Autodesk Inventor part; units mm, degrees
ref_plane "YZ Plane" through (0, 0, 0) normal (1, 0, 0) x (0, 1, 0)
ref_plane "XZ Plane" through (0, 0, 0) normal (0, 1, 0) x (-1, 0, 0)
ref_plane "XY Plane" through (0, 0, 0) normal (0, 0, 1) x (1, 0, 0)
sketch "スケッチ1" plane through (0, 0, 0) normal (1, 0, 0) x (0, 1, 0)
  line L0 (0, 0) -> (1.25, 0)
  line L1 (1.25, 0) -> (1.25, -10)
  line L2 (1.25, -10) -> (0, -10)
  line L3 (0, -10) -> (0, 0)
  line L4 (0, -10) -> (2.25, -10)
  line L5 (2.25, -10) -> (2.25, -12.5)
  line L6 (2.25, -12.5) -> (0, -12.5)
  line L7 (0, -12.5) -> (0, -10)
  line L8 (2.25, -12.3) -> (2.05, -12.5)
  line L9 (1.25, -0.12) -> (1.13, 0)
  point P0 (2.25, -11.25)
  point P1 (1.25, -10)
  dimension "d0" = 45
  dimension "d1" = 2.25
  dimension "d2" = 2.5
  dimension "d3" = 10
  dimension "d7" = 1.25
  dimension "d10" = 45
  dimension "d11" = 0.2
  dimension "d12" = 0.12
revolve "回転1" add sketch "スケッチ1" angle 360 about axis through (0, 0, -10) along (0, 0, 1) contours L0 L9 L1 L2 L3 | L2 L4 L5 L8 L6 L7
thread "ねじ2"
properties part number "CSH-316L-M2_5-10" material "ステンレス鋼"
CAD build for the part. Positions are in the model's coordinates, mm. A direction names the side the tool comes from. Coordinates: 2 decimals unless noted, no trailing zeros. Order: outer loops, then holes, each group sorted by start corner. A loop starts at its lowest first (then second) coordinate and runs counter-clockwise, first axis right, second up. Notation, with made-up numbers: (-2, -34) - (32, -34) arc R16 cw to (32, -14) - close; hole circle Ø6 at (-12, 20.5). An arc over 180 degrees is marked (long way). Answer in a Markdown table with one row per item.
1. 3-axis set-ups, long thin cutter, end or side, ignore diameter. For faces 3 (the face through (0, 0, -12.5)), 4 (the face through (-1.22, -0.27, -5.13)): which of +Z, -Z, +X, -X, +Y, -Y reach the whole face in a straight line?
Answer:
| item | result |
|---|---|
| face 3 | -Z, +X, -X, +Y, -Y |
| face 4 | +Z |
2. Slice it at C-C, the plane z = -5.75. List the corners of the cut face in (x, y), then the cut area to 3 significant figures.
Answer:
| item | result |
|---|---|
| outline | circle Ø2.5 at (0, 0) |
| area | 4.91 mm² |
3. Slice it at A-A, the plane x = 0. List the corners of the cut face in (y, z).
Answer:
| item | result |
|---|---|
| outline | (-2.25, -12.3) - (-2.05, -12.5) - (2.05, -12.5) - (2.25, -12.3) - (2.25, -10) - (1.25, -10) - (1.25, -0.12) - (1.13, 0) - (-1.13, 0) - (-1.25, -0.12) - (-1.25, -10) - (-2.25, -10) - close |
4. Pull direction X, two halves, no side cores. Call faces 1 (the face through (2.23, -0.29, -11.17)), 2 (the face through (0, 0, 0)): +X half, -X half, draft (parallel to the pull), parting line (faces both ways), or undercut.
Answer:
| item | result |
|---|---|
| face 1 | parting line |
| face 2 | draft |
5. Drill centre lines: L1, parallel to Z at x = 1.5, y = 1.15; L2, parallel to Y at x = -0.4, z = -10.75; L3, parallel to Y at x = -1.1, z = -2. Where is each one in solid material? Low to high. Write a range as from..to.
Answer:
| item | result |
|---|---|
| L1 | -12.5..-10 |
| L2 | -2.21..2.21 |
| L3 | -0.59..0.59 |
6. Flat gauge pins, fed straight in: P1, Ø2, axis at x = -0.5, y = 1.5, coming from the +Z side; P2, Ø1, axis at y = 1, z = -11, coming from the +X side; P3, Ø2, axis at x = -0.5, z = -8, coming from the -Y side. Where does each tip first touch, or does it go through?
Answer:
| item | result |
|---|---|
| P1 | z = 0 |
| P2 | x = 2.19 |
| P3 | y = -1.25 |
